from build123d import *

# Parameters (mm, degrees)
SKETCH_1_R                     = 2.25
EXTRUDE_1_DEPTH                = 18
SKETCH_2_R                     = 1.5
CUT_EXTRUDE_1_DEPTH            = 130.976921028
CHAMFER_1_SIZE                 = 1.65
CHAMFER_2_SIZE                 = 2
CUT_EXTRUDE_2_DEPTH            = 10
HOLE_WIZARD_M3_1_D             = 2.5
HOLE_WIZARD_M3_1_CSINK_D       = 3.05
HOLE_WIZARD_M3_1_CSINK_ANGLE   = 90
CHAMFER_3_SIZE                 = 1.65
SKETCH_9_R                     = 2
CUT_EXTRUDE_3_DEPTH            = 133.747881353
CHAMFER_4_SIZE                 = 20
FILLET_1_R                     = 2
CUT_EXTRUDE_4_DEPTH            = 4
FILLET_2_R                     = 2
EXTRUDE_2_DEPTH                = 4
FILLET_3_R                     = 3
FILLET_4_R                     = 3
HOLE_WIZARD_M2_5_1_D           = 2.05
HOLE_WIZARD_M2_5_1_CSINK_D     = 2.55
HOLE_WIZARD_M2_5_1_CSINK_ANGLE = 90
SKETCH_15_W                    = 68.43860018
SKETCH_15_H                    = 10
CUT_EXTRUDE_5_DEPTH            = 87.446064633
FILLET_5_R                     = 2


with BuildPart() as part:
    # 草图1 → 凸台-拉伸1 (new body)
    with BuildSketch(Plane(origin=(0, 0, 0), x_dir=(1, 0, 0), z_dir=(0, 1, 0))):
        Polygon((0, 0), (0, 93), (-4, 93), (-4, 71), (-12, 71), (-12, 62.911688245), (-62.911688245, 12), (-71, 12), (-71, 4), (-93, 4), (-93, 0), align=None)
        with Locations(Location((-8.5, 67.5, 0), (0, 0, 270))):
            Circle(SKETCH_1_R, mode=Mode.SUBTRACT)
        with Locations(Location((-67.5, 8.5, 0), (0, 0, 90))):
            Circle(SKETCH_1_R, mode=Mode.SUBTRACT)
    extrude(amount=EXTRUDE_1_DEPTH)

    # 草图2 → 切除-拉伸1 (cut, through all)
    with BuildSketch(Plane(origin=(0, 0, -4), x_dir=(-1, 0, 0), z_dir=(0, 0, -1))):
        with Locations((73.5, 14)):
            Circle(SKETCH_2_R)
        with Locations((88.5, 14)):
            Circle(SKETCH_2_R)
        with Locations((88.5, 4)):
            Circle(SKETCH_2_R)
        with Locations((73.5, 4)):
            Circle(SKETCH_2_R)
    cut_extrude_1 = extrude(amount=-CUT_EXTRUDE_1_DEPTH, mode=Mode.SUBTRACT)

    # 镜向2: 切除-拉伸1 across plane
    add(cut_extrude_1.mirror(Plane(origin=(0, 0, 0), x_dir=(0.7071067811865513, 0, 0.7071067811865437), z_dir=(0.7071067811865437, 0, -0.7071067811865513))), mode=Mode.SUBTRACT)

    # 倒角1
    chamfer_1_edges = [part.edges().sort_by_distance(p)[0] for p in [
        (-72, 4, 0),
        (-87, 4, 0),
        (-87, 14, 0),
        (-72, 14, 0),
        (0, 4, -72),
        (0, 4, -87),
        (0, 14, -87),
        (0, 14, -72),
    ]]
    chamfer(chamfer_1_edges, length=CHAMFER_1_SIZE)

    # 倒角2
    chamfer_2_edges = [part.edges().sort_by_distance(p)[0] for p in [
        (-71, 9, -12),
        (-12, 9, -71),
    ]]
    chamfer(chamfer_2_edges, length=CHAMFER_2_SIZE)

    # 草图3 → 切除-拉伸2 (cut)
    with BuildSketch(Plane.XZ):
        Polygon((0, 0), (-66.426406871, 0), (0, -66.426406871), align=None)
    extrude(amount=-CUT_EXTRUDE_2_DEPTH, mode=Mode.SUBTRACT)

    # M3 螺纹孔1 (through all)
    with Locations(Plane(origin=(-40.5, 0, -40.5), x_dir=(-0.7071067811865498, 0, 0.7071067811865452), z_dir=(-0.7071067811865452, 0, -0.7071067811865498))):
        with Locations((-41.71930009, 4), (41.71930009, 4)):
            CounterSinkHole(HOLE_WIZARD_M3_1_D / 2, HOLE_WIZARD_M3_1_CSINK_D / 2, counter_sink_angle=HOLE_WIZARD_M3_1_CSINK_ANGLE)

    # 倒角3
    chamfer_3_edges = [part.edges().sort_by_distance(p)[0] for p in [
        (-63.597086912, 4, -2.829319959),
        (-4.597086912, 4, -61.829319959),
    ]]
    chamfer(chamfer_3_edges, length=CHAMFER_3_SIZE)

    # 草图9 → 切除-拉伸3 (cut, through all)
    with BuildSketch(Plane(origin=(0, 18, 0), x_dir=(1, 0, 0), z_dir=(0, 1, 0))):
        with Locations(Location((-52, 4, 0), (0, 0, 270))):
            Circle(SKETCH_9_R)
        with Locations(Location((-40, 4, 0), (0, 0, 270))):
            Circle(SKETCH_9_R)
        with Locations(Location((-4, 40, 0), (0, 0, 90))):
            Circle(SKETCH_9_R)
        with Locations(Location((-4, 52, 0), (0, 0, 90))):
            Circle(SKETCH_9_R)
    extrude(amount=-CUT_EXTRUDE_3_DEPTH, mode=Mode.SUBTRACT)

    # 倒角4
    chamfer_4_edges = [part.edges().sort_by_distance(p)[0] for p in [
        (0, 14, 0),
    ]]
    chamfer(chamfer_4_edges, length=CHAMFER_4_SIZE)

    # 圆角1
    fillet_1_edges = [part.edges().sort_by_distance(p)[0] for p in [
        (-62.911688245, 9, -12),
        (-12, 9, -62.911688245),
    ]]
    fillet(fillet_1_edges, radius=FILLET_1_R)

    # 草图10 → 切除-拉伸4 (cut)
    with BuildSketch(Plane.XZ.offset(-10)):
        Polygon((-58.926406871, -7.5), (-16.742640687, -7.5), (-7.5, -16.742640687), (-7.5, -58.926406871), align=None)
    extrude(amount=-CUT_EXTRUDE_4_DEPTH, mode=Mode.SUBTRACT)

    # 圆角2
    fillet_2_edges = [part.edges().sort_by_distance(p)[0] for p in [
        (-7.5, 12, -58.926406871),
        (-58.926406871, 12, -7.5),
        (-16.742640687, 12, -7.5),
        (-7.5, 12, -16.742640687),
    ]]
    fillet(fillet_2_edges, radius=FILLET_2_R)

    # 草图11 → 凸台-拉伸2 (add)
    with BuildSketch(Plane(origin=(0, 18, 0), x_dir=(1, 0, 0), z_dir=(0, 1, 0))):
        Polygon((-51.597979746, 23.313708499), (-51.597979746, 37.455844123), (-37.455844123, 51.597979746), (-23.313708499, 51.597979746), align=None)
    extrude(amount=-EXTRUDE_2_DEPTH)

    # 圆角3
    fillet_3_edges = [part.edges().sort_by_distance(p)[0] for p in [
        (-23.313708499, 16, -51.597979746),
        (-51.597979746, 16, -23.313708499),
        (-51.597979746, 16, -37.455844123),
        (-37.455844123, 16, -51.597979746),
    ]]
    fillet(fillet_3_edges, radius=FILLET_3_R)

    # 圆角4
    fillet_4_edges = [part.edges().sort_by_distance(p)[0] for p in [
        (0, 14, -20),
        (-20, 14, 0),
    ]]
    fillet(fillet_4_edges, radius=FILLET_4_R)

    # M2.5 螺纹孔1 (through all)
    with Locations(Plane(origin=(0, 18, 0), x_dir=(1, 0, 0), z_dir=(0, 1, 0))):
        with Locations((-45.771419869, 13.272792206), (-17.310371927, 17.310371927), (-40.991378029, 40.991378029), (-13.272792206, 45.771419869)):
            CounterSinkHole(HOLE_WIZARD_M2_5_1_D / 2, HOLE_WIZARD_M2_5_1_CSINK_D / 2, counter_sink_angle=HOLE_WIZARD_M2_5_1_CSINK_ANGLE)

    # 草图15 → 切除-拉伸5 (cut, through all)
    with BuildSketch(Plane(origin=(-33.213203436, 0, -33.213203436), x_dir=(0.7071067811865476, 0, -0.7071067811865475), z_dir=(0.7071067811865475, 0, 0.7071067811865476))):
        with Locations((0, 5)):
            Rectangle(SKETCH_15_W, SKETCH_15_H)
    extrude(amount=-CUT_EXTRUDE_5_DEPTH, mode=Mode.SUBTRACT)

    # 圆角5
    # the kernel refuses this fillet: 2 mm, written as the material it takes off along each edge
    with BuildSketch(Plane(origin=(-61.652543264, 10, -13.259144982), x_dir=(-0.7397286230240017, 0, 0.6729053159836194), z_dir=(0, -1, 0)), Plane(origin=(-13.259144982, -4.650863848, -61.652543264), x_dir=(0.6729053159836488, 0, -0.7397286230239748), z_dir=(0, 1, 0))) as fillet_5_piece_1:
        with BuildLine():
            CenterArc((1.909862491, -1.95277003), FILLET_5_R, 102.476415923, 74.815280531)
            Line((-0.087903584, -1.858267603), (-0.287680192, -1.848817361))
            Line((-0.287680192, -1.848817361), (-0.199776608, 0.009450243))
            Line((-0.199776608, 0.009450243), (0.009450243, 0.199776608))
            ThreePointArc((0.009450243, 0.199776608), (0.960659375, 0.154780563), (1.434579479, 0.195277003))
            Line((1.434579479, 0.195277003), (1.477787025, 0))
        make_face()
    extrude(amount=14.650863848, mode=Mode.SUBTRACT)
    with BuildSketch(Plane(origin=(-57.409902577, 10, -9.016504294), x_dir=(-0.7071067811865462, 0, -0.7071067811865489), z_dir=(0, -1, 0))) as fillet_5_piece_2:
        with BuildLine():
            CenterArc((FILLET_5_R, -FILLET_5_R), FILLET_5_R, 90, 90)
            Line((0, -FILLET_5_R), (0, 0))
            Line((0, 0), (FILLET_5_R, 0))
        make_face()
    extrude(amount=15, mode=Mode.SUBTRACT)
    with BuildSketch(Plane(origin=(-9.016504294, -5, -57.409902577), x_dir=(0.7071067811865487, 0, -0.7071067811865465), z_dir=(0, 1, 0))) as fillet_5_piece_3:
        with BuildLine():
            CenterArc((FILLET_5_R, FILLET_5_R), FILLET_5_R, 180, 90)
            Line((0, FILLET_5_R), (0, 0))
            Line((0, 0), (FILLET_5_R, 0))
        make_face()
    extrude(amount=15, mode=Mode.SUBTRACT)


solid = part.part
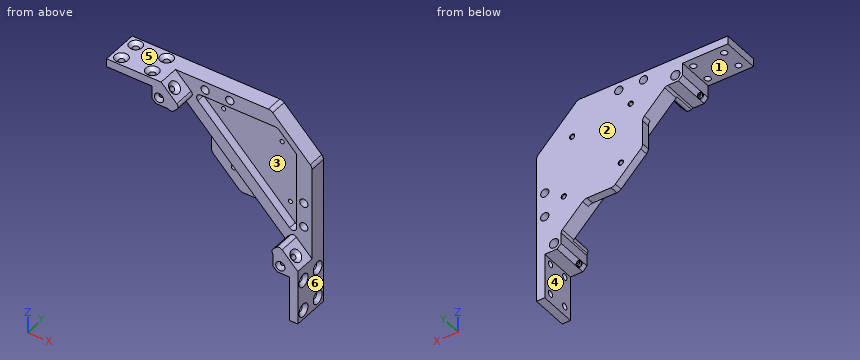
Design review of the part built by this model. Coordinates are the model's own, in mm. Face numbers are marked on the shaded views. A direction names the side the tool comes from. Coordinates: 2 decimals unless noted, no trailing zeros. Write each loop counter-clockwise with the first axis right and the second up, starting at its lowest first coordinate (ties: lowest second). Pieces come first, ordered by that corner, then holes. Notation, with made-up numbers: (18.25, 35.5) -> (58.25, 35.5) arc R16 ccw to (58.25, 49.5) -> close; hole circle Ø4 at (40, 10.5). An arc over 180 degrees is marked (long way). Write each question's results on one line, items separated by ' | '. Start each with the question number.
(1) Take a section at A-A on y = 8.75. Write out the cut boundary in (x, z), and give its area (3 significant figures).
(2) Take a section at C-C on z = -27. Write out the cut boundary in (x, y), and give its area (3 significant figures).
(3) The part is to be moulded in two halves that separate along X. For the marked faces 3, 4, 5 and 6, say which applies: pulls with the +X half, pulls with the -X half, needs draft (parallel to the pull), parting line crosses it, or undercut.
(4) For line 1 along Z through (x, y) = (-2.75, 4); line 2 along Y through (x, z) = (-73.5, -3.05); line 3 along Z through (x, y) = (-2.45, 14), list the stretches that pass through material, from the lowest coordinate up. Write a range as from..to.
(5) Take a section at B-B on z = -88.5. Write out the cut boundary in (x, y).
(6) Clearance check with flat-ended pins moving along their axes: P1, Ø9, axis at y = 5.5, z = -80.5, coming from the -X side; P2, Ø4, axis at x = -61, y = 3, coming from the -Z side; P3, Ø1.5, axis at y = 13, z = -36.5, coming from the -X side. State where each tip first meets the part, or that it passes through.
(7) Tool access review of the marked faces 1 and 2: name each direction out of +Z, -Z, +X, -X, +Y, -Y from which nothing blocks a thin tool from reaching the whole face with its end or side.
Results found:
1) outline: (-93, -4) -> (-71, -4) -> (-71, -10) -> (-69, -12) -> (-63.74, -12) arc R2 cw to (-62.75, -12.26) arc R2 ccw to (-60.34, -11.94) -> (-58.82, -10.43) arc R2 ccw to (-58.82, -7.6) -> (-66.43, 0) -> (-93, 0) -> close; (-12.26, -62.75) arc R2 cw to (-12, -63.74) -> (-12, -69) -> (-10, -71) -> (-4, -71) -> (-4, -93) -> (0, -93) -> (0, -66.43) -> (-7.6, -58.82) arc R2 ccw to (-10.43, -58.82) -> (-11.94, -60.34) arc R2 ccw to start; hole circle Ø4.5 at (-67.5, -8.5); hole circle Ø4.5 at (-8.5, -67.5) | area: 376 mm2
2) outline: (-51.6, 14) -> (-47.91, 14) -> (-47.91, 10) -> (-39.43, 10) -> (-39.43, 14) -> (-7.5, 14) -> (-7.5, 10) -> (0, 10) -> (0, 18) -> (-51.6, 18) -> close | area: 270 mm2
3) face 3: undercut | face 4: pulls with the -X half | face 5: needs draft | face 6: pulls with the +X half
4) line 1: z = -93..-90, -87..-75, -72..-64.76 | line 2: y = 0..2.5, 5.5..12.5, 15.5..18 | line 3: z = -93..-90, -87..-75, -72..-53.26, -50.74..-41.26, -38.74..-17.55
5) outline: (-4, 0) -> (0, 0) -> (0, 0.85) -> (-1.65, 2.5) -> (-4, 2.5) -> close; (-4, 5.5) -> (-1.65, 5.5) -> (0, 7.15) -> (0, 10.85) -> (-1.65, 12.5) -> (-4, 12.5) -> close; (-4, 15.5) -> (-1.65, 15.5) -> (0, 17.15) -> (0, 18) -> (-4, 18) -> close
6) P1: stops at x = -4 | P2: stops at z = -12.53 | P3: stops at x = -39.16
7) face 1: -Z, -X, +Y, -Y | face 2: +Z, -Z, +X, -X, +Y
